```python
from build123d import *

# Parameters (mm, degrees)
SKETCH2_W           = 18
SKETCH2_H           = 3.5
BOSS_EXTRUDE1_DEPTH = 1
SKETCH3_R           = 0.7
CUT_EXTRUDE1_DEPTH  = 2
FILLET1_R           = 0.5
SKETCH4_OUTSIDE_W   = 23.672
SKETCH4_OUTSIDE_H   = 9.172
SKETCH4_OUTSIDE_R   = 1.164013777
CUT_EXTRUDE3_DEPTH  = 2


with BuildPart() as part:
    # Sketch2 → Boss-Extrude1 (new body)
    with BuildSketch(Plane.XY):
        Rectangle(SKETCH2_W, SKETCH2_H)
    extrude(amount=BOSS_EXTRUDE1_DEPTH)

    # Sketch3 → Cut-Extrude1 (cut, through all)
    with BuildSketch(Plane.XY.offset(1)):
        with Locations((-5.3, 0)):
            Circle(SKETCH3_R)
    extrude(amount=-CUT_EXTRUDE1_DEPTH, mode=Mode.SUBTRACT)

    # Fillet1
    fillet1_edges = [part.edges().sort_by_distance(p)[0] for p in [
        (-9, -1.75, 0.5),
        (-9, 1.75, 0.5),
    ]]
    fillet(fillet1_edges, radius=FILLET1_R)

    # Sketch4 outside → Cut-Extrude3 (cut, through all)
    with BuildSketch(Plane(origin=(0, 0, 0), x_dir=(-1, 0, 0), z_dir=(0, 0, -1))):
        Rectangle(SKETCH4_OUTSIDE_W, SKETCH4_OUTSIDE_H)
        with BuildLine():
            Line((-9, -1.75), (8.5, -1.75))
            ThreePointArc((8.5, -1.75), (8.853553391, -1.603553391), (9, -1.25))
            Line((9, -1.25), (9, 1.25))
            ThreePointArc((9, 1.25), (8.853553391, 1.603553391), (8.5, 1.75))
            Line((8.5, 1.75), (-9, 1.75))
            Line((-9, 1.75), (-9, -1.75))
        make_face(mode=Mode.SUBTRACT)
        with Locations((-3.7, 0)):
            Circle(SKETCH4_OUTSIDE_R)
    extrude(amount=-CUT_EXTRUDE3_DEPTH, mode=Mode.SUBTRACT)


solid = part.part
```
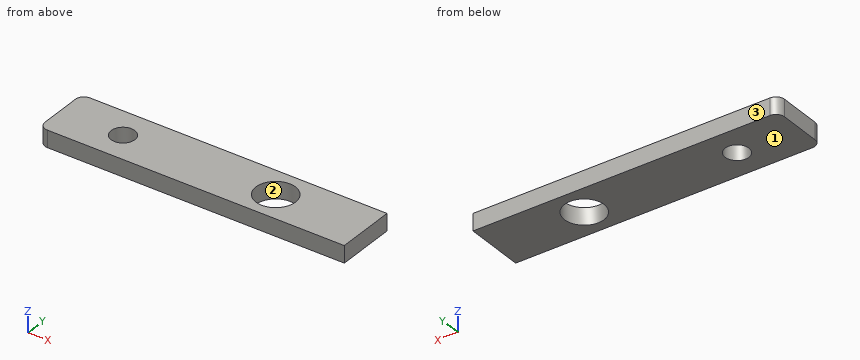
Could you check a few things on this model? Use its own coordinates, in mm. Face numbers are marked on the shaded views. Round coordinates to 2 decimals unless told otherwise and drop trailing zeros. Loops run counter-clockwise (first coordinate to the right, second up) from the corner with the lowest first, then second, coordinate; pieces in that order, holes last. Notation, with made-up numbers: (67, 13) - (120, 13) arc R17 cw to (120, 33) - close; hole circle Ø1 at (4.25, 23.25). An arc over 180 degrees is marked (long way). Answer in a Markdown table with one row per item. Add a question column.
(1) If we section it at B-B (y = 0): Please give me the cut outline in (x, z), plus the area to 3 significant figures.
(2) If we section it at C-C (z = 0.7): Please give me the cut outline in (x, y).
(3) If we mould it in two halves opening along Y, with no side actions, what happens to the marked faces 1, 2 and 3? For each: pulls with the +Y half, pulls with the -Y half, needs draft (parallel to the pull), parting line crosses it, or undercut.
(4) I need wall thicknesses on line 1 along Y through (x, z) = (-5.3, 0.7); line 2 along Y through (x, z) = (3.7, 0.3); line 3 along X through (y, z) = (-0.15, 0.4). Which ranges of each line are inside material? Lowest first, please.
(5) If we section it at D-D (y = -0.95): Please give me the cut outline in (x, z), plus the area to 3 significant figures.
(6) If we section it at A-A (x = -5.3): Please give me the cut outline in (y, z), plus the area to 3 significant figures.
Model answer:
| question | item | result |
|---|---|---|
| 1 | outline | (-9, 0) - (-6, 0) - (-6, 1) - (-9, 1) - close; (-4.6, 0) - (2.54, 0) - (2.54, 1) - (-4.6, 1) - close; (4.86, 0) - (9, 0) - (9, 1) - (4.86, 1) - close |
| 1 | area | 14.3 mm² |
| 2 | outline | (-9, -1.25) arc R0.5 ccw to (-8.5, -1.75) - (9, -1.75) - (9, 1.75) - (-8.5, 1.75) arc R0.5 ccw to (-9, 1.25) - close; hole circle Ø1.4 at (-5.3, 0); hole circle Ø2.33 at (3.7, 0) |
| 3 | face 1 | needs draft |
| 3 | face 2 | undercut |
| 3 | face 3 | pulls with the +Y half |
| 4 | line 1 | y = -1.75 to -0.7, 0.7 to 1.75 |
| 4 | line 2 | y = -1.75 to -1.16, 1.16 to 1.75 |
| 4 | line 3 | x = -9 to -5.98, -4.62 to 2.55, 4.85 to 9 |
| 5 | outline | (-9, 0) - (3.03, 0) - (3.03, 1) - (-9, 1) - close; (4.37, 0) - (9, 0) - (9, 1) - (4.37, 1) - close |
| 5 | area | 16.7 mm² |
| 6 | outline | (-1.75, 0) - (-0.7, 0) - (-0.7, 1) - (-1.75, 1) - close; (0.7, 0) - (1.75, 0) - (1.75, 1) - (0.7, 1) - close |
| 6 | area | 2.10 mm² |
